Could you check a few things on this model? Use its own coordinates, in mm. Give positions to 0.01 mm unless a question says otherwise; leave off trailing zeros. Write each loop counter-clockwise with the first axis right and the second up, starting at its lowest first coordinate (ties: lowest second). Pieces come first, ordered by that corner, then holes. Notation, with made-up numbers: (16, -36.75) - (30, -36.75) arc R4 ccw to (30, -31.75) - close; hole circle Ø11 at (-25, 72). An arc over 180 degrees is marked (long way). Use one line per item in the form item = value.
Autodesk Inventor part; units mm, degrees
ref_plane "YZ Plane" through (0, 0, 0) normal (1, 0, 0) x (0, 1, 0)
ref_plane "XZ Plane" through (0, 0, 0) normal (0, 1, 0) x (-1, 0, 0)
ref_plane "XY Plane" through (0, 0, 0) normal (0, 0, 1) x (1, 0, 0)
sketch "Sketch1" plane through (0, 0, 0) normal (0, 0, 1) x (1, 0, 0)
  line L0 (65.8846, 0) -> (24.1154, 24.1154)
  line L1 (24.1154, 24.1154) -> (0, 65.8846)
  line L2 (0, 65.8846) -> (0, 114.1154)
  line L3 (0, 114.1154) -> (24.1154, 155.8846)
  line L4 (24.1154, 155.8846) -> (65.8846, 180)
  line L5 (65.8846, 180) -> (114.1154, 180)
  line L6 (114.1154, 180) -> (155.8846, 155.8846)
  line L7 (155.8846, 155.8846) -> (180, 114.1154)
  line L8 (180, 114.1154) -> (180, 65.8846)
  line L9 (180, 65.8846) -> (155.8846, 24.1154)
  line L10 (155.8846, 24.1154) -> (114.1154, 0)
  line L11 (114.1154, 0) -> (65.8846, 0)
  line L12 (70, 70) -> (110, 70)
  line L13 (110, 70) -> (110, 110)
  line L14 (110, 110) -> (70, 110)
  line L15 (70, 110) -> (70, 70)
  circle A0 centre (90, 150) radius 10
  circle A1 centre (47.5736, 132.4264) radius 10
  circle A2 centre (132.4264, 132.4264) radius 10
  circle A3 centre (150, 90) radius 10
  circle A4 centre (30, 90) radius 10
  circle A5 centre (47.5736, 47.5736) radius 10
  circle A6 centre (90, 30) radius 10
  circle A7 centre (132.4264, 47.5736) radius 10
  point P0 (0, 0)
  point P1 (90, 90)
  point P2 (90, 90)
  dimension "d1" = 20
  dimension "d2" = 20
extrude "Extrusion1" add sketch "Sketch1" along normal blind 6
properties part number "P2-11"
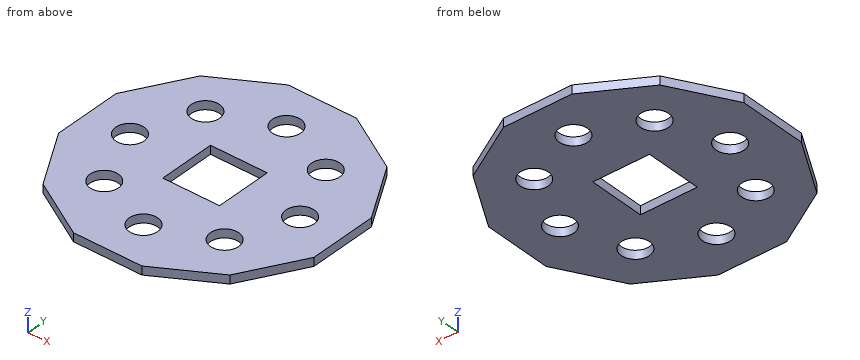
1. Imagine slicing it at D-D, the plane z = 3. State how many separate pieces and enclosed holes the cut face has, and give its area (3 significant figures).
Response values:
separate_pieces = 1
enclosed_holes = 9
area = 21,900 mm²
2. If I drill on line 1 (Y direction, x = 90, z = 3.05); line 2 (X direction, y = 44, z = 5.65); line 3 (Y direction, x = 109, z = 4.2), over which ranges is the centre line in solid material (lowest first)? Write a range as from..to.
Response values:
line_1 = 0..20, 40..70, 110..140, 160..180
line_2 = 12.64..38.23, 56.91..123.09, 141.77..167.36
line_3 = 0..70, 110..180
3. For pin 1 (3 mm diameter, centred on y = 53, z = 1.5, fed in from +X), with a flat end and sliding along its axis, tell me the tip position at first contact or that it passes through.
Response values:
pin_1 = 173.43
4. Imagine slicing it at A-A, the plane y = 90. List the corners of the cut face in (x, z) for me.
Response values:
outline = (0, 0) - (20, 0) - (20, 6) - (0, 6) - close; (40, 0) - (70, 0) - (70, 6) - (40, 6) - close; (110, 0) - (140, 0) - (140, 6) - (110, 6) - close; (160, 0) - (180, 0) - (180, 6) - (160, 6) - close
5. Imagine slicing it at B-B, the plane x = 30. List the corners of the cut face in (y, z) for me.
Response values:
outline = (20.72, 0) - (80, 0) - (80, 6) - (20.72, 6) - close; (100, 0) - (159.28, 0) - (159.28, 6) - (100, 6) - close
